CAD build for the part. Positions are in the model's coordinates, mm. A direction names the side the tool comes from. Give positions to 0.01 mm unless a question says otherwise; leave off trailing zeros. Write each loop counter-clockwise with the first axis right and the second up, starting at its lowest first coordinate (ties: lowest second). Pieces come first, ordered by that corner, then holes. Notation, with made-up numbers: (-30, -15) - (-10, -15) arc R25 ccw to (-10, 14) - close; hole circle Ø6 at (29, 48.5). An arc over 180 degrees is marked (long way). Put each result on its own line as item: value. Start each with the question number.
1. Cut at C-C on y = 1.35. Give the number of separate pieces and of enclosed holes in the cut face, and give its area (3 significant figures).
2. Tool access for faces 1 (the flat face through (105, 1, -38)), 2 (the flat face through (112, 1, -49.5)), 3 (the flat face through (10, 1, -36.5)): list every direction of +Z, -Z, +X, -X, +Y, -Y with a clear straight run to the whole face (end or side of a thin tool).
3. Drop flat-ended pins along their axis: pin 1 (0.9 mm diameter, centred on y = 1, z = -58, fed in from +X); pin 2 (1.2 mm diameter, centred on x = 16.5, z = -30.5, fed in from -Y); pin 3 (1.5 mm diameter, centred on y = 1, z = -65, fed in from -X); pin 4 (4 mm diameter, centred on x = 46, z = -43.5, fed in from -Y). Give the stop position or say it passes through.
4. Cut at B-B on x = 55. List the corners of the cut face in (y, z).
5. Mould opens along X. For faces 4 (the flat face through (100, 1, -33.5)), 5 (the flat face through (110, 1, -38)), 6 (the flat face through (50.5, 1, -65)), 7 (the flat face through (-3, 1, -45)) say: +X half, -X half, draft (parallel to the pull), parting line (faces both ways), or undercut.
6. Cut at D-D on z = -54. List the corners of the cut face in (x, y).
7. Cut at A-A on z = -65.5. List the corners of the cut face in (x, y), and give its area (3 significant figures).
8. Wall check: line 1 (X direction, y = 1.4, z = -65.5); line 2 (X direction, y = 2.45, z = -37); line 3 (Z direction, x = 93.5, y = 1.2). Give the ranges that are in metal, low to high.
from build123d import *

# Parameters (mm, degrees)
SKETCH1_R           = 0.75
SKETCH1_W           = 10.1
SKETCH1_H           = 3.1
SKETCH1_R_2         = 1.5
BOSS_EXTRUDE1_DEPTH = 3
FILLET1_R           = 3


with BuildPart() as part:
    # Sketch1 → Boss-Extrude1 (new body)
    with BuildSketch(Plane(origin=(0, 0, 0), x_dir=(1, 0, 0), z_dir=(0, 1, 0))):
        Polygon((0, 20.5), (0, 0), (110, 0), (110, 20.5), (113, 20.5), (113, 30.5), (110, 30.5), (110, 33.5), (107, 33.5), (107, 32), (104, 32), (104, 33.5), (95, 33.5), (95, 36.5), (104, 36.5), (104, 38), (107, 38), (107, 36.5), (110, 36.5), (110, 39.5), (113, 39.5), (113, 49.5), (110, 49.5), (110, 70), (0, 70), (0, 49.5), (-3, 49.5), (-3, 39.5), (0, 39.5), (0, 36.5), (3, 36.5), (3, 38), (6, 38), (6, 36.5), (15, 36.5), (15, 33.5), (6, 33.5), (6, 32), (3, 32), (3, 33.5), (0, 33.5), (0, 30.5), (-3, 30.5), (-3, 20.5), align=None)
        with Locations(Location((16.5, 30.5, 0), (0, 0, 270))):
            Circle(SKETCH1_R, mode=Mode.SUBTRACT)
        with Locations(Location((93.5, 30.5, 0), (0, 0, 270))):
            Circle(SKETCH1_R, mode=Mode.SUBTRACT)
        with Locations((45.45, 65.5)):
            Rectangle(SKETCH1_W, SKETCH1_H, mode=Mode.SUBTRACT)
        with Locations(Location((55, 65.5, 0), (0, 0, 270))):
            Circle(SKETCH1_R_2, mode=Mode.SUBTRACT)
        with Locations((64.55, 65.5)):
            Rectangle(SKETCH1_W, SKETCH1_H, mode=Mode.SUBTRACT)
    extrude(amount=BOSS_EXTRUDE1_DEPTH)

    # Fillet1
    fillet1_edges = [part.edges().sort_by_distance(p)[0] for p in [
        (110, 1.5, 0),
        (0, 1.5, 0),
        (0, 1.5, -70),
        (110, 1.5, -70),
    ]]
    fillet(fillet1_edges, radius=FILLET1_R)


solid = part.part
Report:
1. separate pieces: 1
1. enclosed holes: 5
1. area: 7,630 mm²
2. face 1: +Y, -Y
2. face 2: -Z, +X, +Y, -Y
2. face 3: -X, +Y, -Y
3. pin 1: stops at x = 110
3. pin 2: passes through
3. pin 3: stops at x = 0
3. pin 4: stops at y = 0
4. outline: (0, -70) - (3, -70) - (3, -67) - (0, -67) - close; (0, -64) - (3, -64) - (3, 0) - (0, 0) - close
5. face 4: draft
5. face 5: +X half
5. face 6: undercut
5. face 7: -X half
6. outline: (0, 0) - (110, 0) - (110, 3) - (0, 3) - close
7. outline: (0, 0) - (40.4, 0) - (40.4, 3) - (0, 3) - close; (50.5, 0) - (53.5, 0) - (53.5, 3) - (50.5, 3) - close; (56.5, 0) - (59.5, 0) - (59.5, 3) - (56.5, 3) - close; (69.6, 0) - (110, 0) - (110, 3) - (69.6, 3) - close
7. area: 260 mm²
8. line 1: x = 0 to 40.4, 50.5 to 53.5, 56.5 to 59.5, 69.6 to 110
8. line 2: x = 0 to 3, 6 to 104, 107 to 110
8. line 3: z = -70 to -31.25, -29.75 to 0
